Verification items for this drawing (mm, ordinates from the low corner). Give positions to 0.01 mm unless a question says otherwise; leave off trailing zeros. Loops run counter-clockwise (first coordinate to the right, second up) from the corner with the lowest first, then second, coordinate; pieces in that order, holes last. Notation, with made-up numbers: (76.5, 11) -> (110.5, 11) arc R6 ccw to (110.5, 20) -> close; hole circle Ø7 at (-7.75, 8.25). An arc over 180 degrees is marked (long way). Answer in a Markdown table with one row per item. Add a question column.
Q1. Gauge pin test, flat ends, axial feed: P1, Ø12, axis at y = 35.5, z = 364.5, coming from the -X side; P2, Ø12, axis at x = 850, y = 14.5, coming from the +Z side. Record the tip position at first contact, or that the pin passes through.
Q2. Section check B-B on z = 298. Enter the section's corners in (x, y), and give its area (3 significant figures).
Q3. Section check C-C on x = 1391. Enter the section's corners in (y, z).
Q4. Material ranges on probe 1 along X at (y, z) = (33.5, 310.5); probe 2 along X at (y, z) = (30.5, 458); probe 3 along Z at (x, y) = (1014, 3.5), recorded low to high.
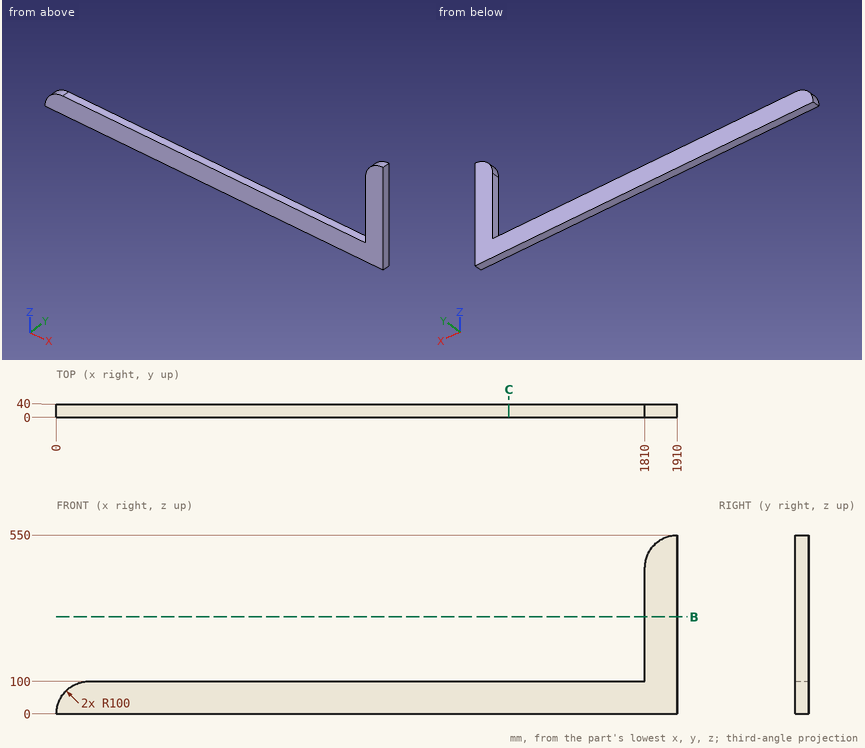
Taken from the geometry:
| question | item | result |
|---|---|---|
| 1 | P1 | stops at x = 1810 |
| 1 | P2 | stops at z = 100 |
| 2 | outline | (1810, 0) -> (1910, 0) -> (1910, 40) -> (1810, 40) -> close |
| 2 | area | 4,000 mm² |
| 3 | outline | (0, 0) -> (40, 0) -> (40, 100) -> (0, 100) -> close |
| 4 | probe 1 | x = 1810 to 1910 |
| 4 | probe 2 | x = 1810.32 to 1910 |
| 4 | probe 3 | z = 0 to 100 |
